Verification items for the finished model (mm, model axes). Face numbers are marked on the shaded views. A direction names the side the tool comes from. Coordinates: 2 decimals unless noted, no trailing zeros. Write each loop counter-clockwise with the first axis right and the second up, starting at its lowest first coordinate (ties: lowest second). Pieces come first, ordered by that corner, then holes. Notation, with made-up numbers: M -13.5,58.25 L 38.5,58.25 A36 cw 38.5,95.25 Z; hole C -21.75,75.5 d11. An arc over 180 degrees is marked long. One line per item, written item: value.
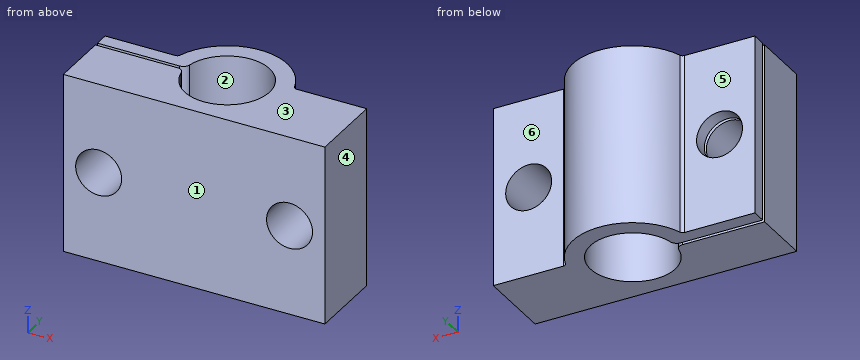
```python
from build123d import *

# Parameters (mm, degrees)
F1_DEPTH = 25.4
F2_R     = 1
F3_R     = 0.5
F4_R     = 3.25
F5_DEPTH = 17.001


with BuildPart() as f1:
    # F0 (on Top) → F1 (new body)
    with BuildSketch(Plane.XY):
        with BuildLine():
            Line((-18.5, -0.25), (-18.5, -8.5))
            Line((-18.5, -8.5), (18.5, -8.5))
            Line((18.5, -8.5), (18.5, 2.25))
            Line((18.5, 2.25), (8.196798, 2.25))
            ThreePointArc((8.196798, 2.25), (0, 8.5), (-8.196798, 2.25))
            Line((-8.196798, 2.25), (-18.5, 2.25))
            Line((-18.5, 2.25), (-18.5, 0.25))
            Line((-18.5, 0.25), (-5.994789, 0.25))
            ThreePointArc((-5.994789, 0.25), (6, 0), (-5.994789, -0.25))
            Line((-5.994789, -0.25), (-18.5, -0.25))
        make_face()
    extrude(amount=F1_DEPTH)

    # F2
    f2_edges = [f1.edges().sort_by_distance(p)[0] for p in [
        (-5.994789, 0.25, 12.7),
        (-5.994789, -0.25, 12.7),
    ]]
    fillet(f2_edges, radius=F2_R)

    # F3
    f3_edges = [f1.edges().sort_by_distance(p)[0] for p in [
        (-8.196798, 2.25, 12.7),
        (8.196798, 2.25, 12.7),
    ]]
    fillet(f3_edges, radius=F3_R)

    # F4 (on face) → F5 (cut, through all)
    with BuildSketch(Plane.XZ.offset(8.5)):
        with Locations((-13.5, 12.7)):
            Circle(F4_R)
        with Locations((13.5, 12.7)):
            Circle(F4_R)
    extrude(amount=-F5_DEPTH, mode=Mode.SUBTRACT)


solid = f1.part
```
Item 1: Cross-section at B-B, the plane x = 0. Enter the section's corners in (y, z), and give its area (3 significant figures).
The answers:
outline: M -8.5,0 L -6,0 L -6,25.4 L -8.5,25.4 Z; M 6,0 L 8.5,0 L 8.5,25.4 L 6,25.4 Z
area: 127 mm²
Item 2: Access from +Z, -Z, +X, -X, +Y, -Y to the whole of each face (thin tool, end or side, straight path). Record for the marked faces 4, 5 and 6.
The answers:
face 4: +Z, -Z, +X, +Y, -Y
face 5: +Z, -Z, -X, +Y
face 6: +Z, -Z, +X, +Y
Item 3: Go/stop test with flat-tipped pins: P1, Ø7.5, axis at x = -13.5, z = 12.7, coming from the +Y side; P2, Ø10.5, axis at x = 13.5, z = 12.7, coming from the +Y side; P3, Ø5, axis at x = -9.5, z = 19, coming from the +Y side. Record where each tip stops, or that it passes through.
The answers:
P1: stops at y = 2.25
P2: stops at y = 2.37
P3: stops at y = 4.82
Item 4: Scan lines: line 1 (Y direction, x = -12, z = 21); line 2 (Z direction, x = 13.5, y = -2.25); line 3 (X direction, y = 1.5, z = 9.75). Record each from-to range of solid material in increasing order.
The answers:
line 1: y = -8.5 to -0.25, 0.25 to 2.25
line 2: z = 0 to 9.45, 15.95 to 25.4
line 3: x = -18.5 to -14.86, -12.14 to -5.81, 5.81 to 12.14, 14.86 to 18.5
Item 5: Cross-section at C-C, the plane y = 5.5. Enter the section's corners in (x, z), and give its area (3 significant figures).
The answers:
outline: M -6.48,0 L -2.4,0 L -2.4,25.4 L -6.48,25.4 Z; M 2.4,0 L 6.48,0 L 6.48,25.4 L 2.4,25.4 Z
area: 207 mm²
Item 6: Cross-section at A-A, the plane z = 12.7. Enter the section's corners in (x, y).
The answers:
outline: M -18.5,-8.5 L -16.75,-8.5 L -16.75,-0.25 L -18.5,-0.25 Z; M -18.5,0.25 L -16.75,0.25 L -16.75,2.25 L -18.5,2.25 Z; M -10.25,-8.5 L 10.25,-8.5 L 10.25,2.25 L 8.57,2.25 A0.5 cw 8.09,2.6 A8.5 ccw -8.09,2.6 A0.5 cw -8.57,2.25 L -10.25,2.25 L -10.25,0.25 L -6.89,0.25 A1 ccw -5.9,1.07 A6 cw long -5.9,-1.07 A1 ccw -6.89,-0.25 L -10.25,-0.25 Z; M 16.75,-8.5 L 18.5,-8.5 L 18.5,2.25 L 16.75,2.25 Z
Item 7: Draft check along Y on the marked faces 1, 2 and 3. Enter one of: released by +Y, released by -Y, zero draft, split by the parting line, or undercut.
The answers:
face 1: released by -Y
face 2: undercut
face 3: zero draft
Item 8: Cross-section at D-D, the plane x = -13.5. Enter the section's corners in (y, z), and give its area (3 significant figures).
The answers:
outline: M -8.5,0 L -0.25,0 L -0.25,9.45 L -8.5,9.45 Z; M -8.5,15.95 L -0.25,15.95 L -0.25,25.4 L -8.5,25.4 Z; M 0.25,0 L 2.25,0 L 2.25,9.45 L 0.25,9.45 Z; M 0.25,15.95 L 2.25,15.95 L 2.25,25.4 L 0.25,25.4 Z
area: 194 mm²
